Part model, mm, in its own coordinate system. A direction names the side the tool comes from. Round coordinates to 2 decimals unless told otherwise and drop trailing zeros. Write each loop counter-clockwise with the first axis right and the second up, starting at its lowest first coordinate (ties: lowest second). Pieces come first, ordered by that corner, then holes.
from build123d import *

# Parameters (mm, degrees)
SKETCH1_W                         = 127
SKETCH1_H                         = 50.8
BOSS_EXTRUDE1_DEPTH               = 6.35
TAPPED_HOLE_FOR_10_32_HELICOIL1_D = 5.1054
SKETCH7_W                         = 127
SKETCH7_H                         = 14.2875
CUT_EXTRUDE2_DEPTH                = 70.560764803
TAPPED_HOLE_FOR_10_32_HELICOIL3_D = 5.1054
SKETCH4_R                         = 4.7625
CUT_EXTRUDE1_DEPTH                = 70.560764803
CUT_EXTRUDE4_DEPTH                = 3.175
F_10_CLEARANCE_HOLE3_D            = 5.1054
F_10_CLEARANCE_HOLE3_DEPTH        = 12.7
F_10_CLEARANCE_HOLE3_TIP          = 1.533816902


with BuildPart() as part:
    # Sketch1 → Boss-Extrude1 (new, symmetric)
    with BuildSketch(Plane(origin=(0, 0, 0), x_dir=(1, 0, 0), z_dir=(0, 1, 0))):
        Rectangle(SKETCH1_W, SKETCH1_H)
    extrude(amount=BOSS_EXTRUDE1_DEPTH, both=True)

    # Tapped Hole for #10-32 Helicoil1 (through all)
    with Locations(Plane(origin=(0, 0, -25.4), x_dir=(-1, 0, 0), z_dir=(0, 0, -1))):
        with Locations((-57.15, 0), (57.15, 0)):
            Hole(TAPPED_HOLE_FOR_10_32_HELICOIL1_D / 2)

    # Sketch7 → Cut-Extrude2 (cut, through all)
    with BuildSketch(Plane(origin=(0, 6.35, 0), x_dir=(1, 0, 0), z_dir=(0, 1, 0))):
        with Locations((0, -18.25625)):
            Rectangle(SKETCH7_W, SKETCH7_H)
    extrude(amount=-CUT_EXTRUDE2_DEPTH, mode=Mode.SUBTRACT)

    # Tapped Hole for #10-32 Helicoil3 (through all)
    with Locations(Plane.XY.offset(11.1125)):
        with Locations((-38.1, 0), (38.1, 0)):
            Hole(TAPPED_HOLE_FOR_10_32_HELICOIL3_D / 2)

    # Sketch4 → Cut-Extrude1 (cut, through all)
    with BuildSketch(Plane(origin=(0, 6.35, 0), x_dir=(1, 0, 0), z_dir=(0, 1, 0))):
        with Locations(Location((-38.1, 0, 0), (0, 0, 270))):
            Circle(SKETCH4_R)
        with Locations(Location((38.1, 0, 0), (0, 0, 270))):
            Circle(SKETCH4_R)
        with Locations(Location((0, 4.7625, 0), (0, 0, 270))):
            Circle(SKETCH4_R)
    extrude(amount=-CUT_EXTRUDE1_DEPTH, mode=Mode.SUBTRACT)

    # Sketch11 → Cut-Extrude4 (cut)
    with BuildSketch(Plane(origin=(0, 6.35, 0), x_dir=(1, 0, 0), z_dir=(0, 1, 0))):
        with BuildLine():
            Line((-22.225, 20.6375), (22.225, 20.6375))
            ThreePointArc((22.225, 20.6375), (26.715128061, 18.777628061), (28.575, 14.2875))
            Line((28.575, 14.2875), (28.575, -11.1125))
            Line((28.575, -11.1125), (-28.575, -11.1125))
            Line((-28.575, -11.1125), (-28.575, 14.2875))
            ThreePointArc((-28.575, 14.2875), (-26.715128061, 18.777628061), (-22.225, 20.6375))
        make_face()
    extrude(amount=-CUT_EXTRUDE4_DEPTH, mode=Mode.SUBTRACT)

    # #10 Clearance Hole3
    with Locations(Plane(origin=(0, 3.175, 0), x_dir=(1, 0, 0), z_dir=(0, 1, 0))):
        with Locations((-23.0124, 4.7625), (23.0124, 4.7625)):
            Hole(F_10_CLEARANCE_HOLE3_D / 2, depth=F_10_CLEARANCE_HOLE3_DEPTH)
            with Locations((0, 0, -(F_10_CLEARANCE_HOLE3_DEPTH + F_10_CLEARANCE_HOLE3_TIP / 2))):  # 118° drill point
                Cone(0, F_10_CLEARANCE_HOLE3_D / 2, F_10_CLEARANCE_HOLE3_TIP, mode=Mode.SUBTRACT)


solid = part.part
Q1. Wall check: line 1 (Y direction, x = -57, z = 2); line 2 (X direction, y = 1, z = -1.5). Give the ranges that are in metal, low to high.
Q2. Drop flat-ended pins along their axis: P1, Ø4, axis at x = -23.01, z = -4.76, coming from the +Y side; P2, Ø3.5, axis at x = 3, y = 5, coming from the +Z side; P3, Ø1.5, axis at x = -1, z = 2.5, coming from the +Y side (3 decimals). Give the stop position or say it passes through.
Q3. Saw through at D-D, the plane z = -13. Write the cut outline in (x, y) (3 decimals).
Q4. Tool access for faces 4 (the cylindrical face through (-2.9, -1.52, -8.54)), 5 (the flat face through (0, 5, -20.638)): list every direction of +Z, -Z, +X, -X, +Y, -Y with a clear straight run to the whole face (end or side of a thin tool).
Q5. Two-plate mould, pull along Z, no slides. Class faces 1 (the cylindrical face through (-25.447, -1.654, -5.529)), 2 (the flat face through (-63.5, 0, -7)), 3 (the flat face through (-1, 0, -25.4)): released by +Z, released by -Z, zero draft, split by the parting line, or undercut.
Q6. Saw through at C-C, the plane z = 2. Write the cut outline in (x, y) (3 decimals), and give its area (3 significant figures).
Q7. Saw through at A-A, the plane y = 0. Give the number of separate pieces and of enclosed holes in the cut face, and give its area (3 significant figures).
Q8. Saw through at B-B, the plane x = 57.15. Write the cut outline in (y, z).
Computed:
1. line 1: y = -6.35 to -2.55, 2.55 to 6.35
1. line 2: x = -63.5 to -59.5, -54.8 to -42.62, -33.58 to -3.47, 3.47 to 33.58, 42.62 to 54.8, 59.5 to 63.5
2. P1: passes through
2. P2: stops at z = -20.64
2. P3: stops at y = 3.175
3. outline: (-63.5, -6.35) - (63.5, -6.35) - (63.5, 6.35) - (28.575, 6.35) - (28.575, 3.175) - (-28.575, 3.175) - (-28.575, 6.35) - (-63.5, 6.35) - close; hole circle Ø5.105 at (-57.15, 0); hole circle Ø5.105 at (-38.1, 0); hole circle Ø5.105 at (38.1, 0); hole circle Ø5.105 at (57.15, 0)
4. face 4: +Y, -Y
4. face 5: +Z, +Y
5. face 1: undercut
5. face 2: zero draft
5. face 3: released by -Z
6. outline: (-63.5, -6.35) - (-42.422, -6.35) - (-42.422, 6.35) - (-63.5, 6.35) - close; (-33.778, -6.35) - (33.778, -6.35) - (33.778, 6.35) - (28.575, 6.35) - (28.575, 3.175) - (-28.575, 3.175) - (-28.575, 6.35) - (-33.778, 6.35) - close; (42.422, -6.35) - (63.5, -6.35) - (63.5, 6.35) - (42.422, 6.35) - close; hole circle Ø5.105 at (-57.15, 0); hole circle Ø5.105 at (57.15, 0)
6. area: 1,170 mm2
7. separate pieces: 5
7. enclosed holes: 3
7. area: 3,730 mm2
8. outline: (-6.35, -25.4) - (-2.55, -25.4) - (-2.55, 11.11) - (-6.35, 11.11) - close; (2.55, -25.4) - (6.35, -25.4) - (6.35, 11.11) - (2.55, 11.11) - close
